Could you check a few things on this model? Use its own coordinates, in mm. A direction names the side the tool comes from. Give positions to 0.01 mm unless a question says otherwise; leave off trailing zeros. Write each loop counter-clockwise with the first axis right and the second up, starting at its lowest first coordinate (ties: lowest second). Pieces come first, ordered by that corner, then holes. Notation, with made-up numbers: (-22.75, 4.25) -> (22.25, 4.25) arc R22 ccw to (22.25, 36.25) -> close; hole circle Ø7 at (-32.75, 78.25). An arc over 180 degrees is marked (long way). One line per question, with ' | ' between items.
from build123d import *

# Parameters (mm, degrees)
SKETCH1_W           = 444.5
SKETCH1_H           = 285.75
BOSS_EXTRUDE1_DEPTH = 25.4
SKETCH2_R           = 6.7437
CUT_EXTRUDE1_DEPTH  = 530.035417056
SKETCH3_R           = 9.525
CUT_EXTRUDE2_DEPTH  = 7.62
SKETCH4_R           = 6.7437
CUT_EXTRUDE3_DEPTH  = 530.035417056


with BuildPart() as part:
    # Sketch1 → Boss-Extrude1 (new body)
    with BuildSketch(Plane.XY):
        with Locations((222.25, 142.875)):
            Rectangle(SKETCH1_W, SKETCH1_H)
    extrude(amount=BOSS_EXTRUDE1_DEPTH)

    # Sketch2 → Cut-Extrude1 (cut, through all)
    with BuildSketch(Plane.XY):
        with Locations((21.4376, 266.7)):
            Circle(SKETCH2_R)
        with Locations((423.0624, 266.7)):
            Circle(SKETCH2_R)
        with Locations((21.4376, 19.05)):
            Circle(SKETCH2_R)
        with Locations((423.0624, 19.05)):
            Circle(SKETCH2_R)
    extrude(amount=CUT_EXTRUDE1_DEPTH, mode=Mode.SUBTRACT)

    # Sketch3 → Cut-Extrude2 (cut)
    with BuildSketch(Plane.XY):
        with Locations(Location((21.4376, 266.7, 0), (0, 0, 180))):
            Circle(SKETCH3_R)
        with Locations(Location((423.0624, 266.7, 0), (0, 0, 180))):
            Circle(SKETCH3_R)
        with Locations(Location((21.4376, 19.05, 0), (0, 0, 180))):
            Circle(SKETCH3_R)
        with Locations(Location((423.0624, 19.05, 0), (0, 0, 180))):
            Circle(SKETCH3_R)
    extrude(amount=CUT_EXTRUDE2_DEPTH, mode=Mode.SUBTRACT)

    # Sketch4 → Cut-Extrude3 (cut, through all)
    with BuildSketch(Plane.XY):
        with Locations((193.675, 114.3)):
            Circle(SKETCH4_R)
        with Locations((371.475, 114.3)):
            Circle(SKETCH4_R)
        with Locations((193.675, 266.7)):
            Circle(SKETCH4_R)
        with Locations((371.475, 266.7)):
            Circle(SKETCH4_R)
    extrude(amount=CUT_EXTRUDE3_DEPTH, mode=Mode.SUBTRACT)


solid = part.part
Q1. Imagine slicing it at A-A on y = 114.3. Please give me the cut outline in (x, z), and give its area (3 significant figures).
Answer below:
outline: (0, 0) -> (186.93, 0) -> (186.93, 25.4) -> (0, 25.4) -> close; (200.42, 0) -> (364.73, 0) -> (364.73, 25.4) -> (200.42, 25.4) -> close; (378.22, 0) -> (444.5, 0) -> (444.5, 25.4) -> (378.22, 25.4) -> close | area: 10,600 mm^2
Q2. If we mould it in two halves opening along Y, with no side actions, what happens to faces 1 (the flat face through (430, 21, 7.62)), 2 (the flat face through (219, 0, 13)), 3 (the flat face through (219, 285.75, 13)), 4 (the cylindrical face through (22.678, 9.606, 3.757))? For each: +Y half, -Y half, draft (parallel to the pull), parting line (faces both ways), or undercut.
Answer below:
face 1: undercut | face 2: -Y half | face 3: +Y half | face 4: undercut
Q3. Imagine slicing it at C-C on y = 19.05. Please give me the cut outline in (x, z), and give its area (3 significant figures).
Answer below:
outline: (0, 0) -> (11.91, 0) -> (11.91, 7.62) -> (14.69, 7.62) -> (14.69, 25.4) -> (0, 25.4) -> close; (28.18, 7.62) -> (30.96, 7.62) -> (30.96, 0) -> (413.54, 0) -> (413.54, 7.62) -> (416.32, 7.62) -> (416.32, 25.4) -> (28.18, 25.4) -> close; (429.81, 7.62) -> (432.59, 7.62) -> (432.59, 0) -> (444.5, 0) -> (444.5, 25.4) -> (429.81, 25.4) -> close | area: 10,500 mm^2
Q4. Will these pins go through, and if not, where does the flat tip stop? pin 1 (21 mm diameter, centred on x = 423.5, y = 269.5, fed in from -Z); pin 2 (15 mm diameter, centred on x = 21.44, y = 266.7, fed in from -Z).
Answer below:
pin 1: stops at z = 0 | pin 2: stops at z = 7.62
Q5. If I drill on line 1 along X through (y, z) = (114.3, 6); line 2 along X through (y, z) = (266.7, 10); line 3 along X through (y, z) = (19.05, 19.5), over which ranges is the centre line in solid material (lowest first)?
Answer below:
line 1: x = 0 to 186.93, 200.42 to 364.73, 378.22 to 444.5 | line 2: x = 0 to 14.69, 28.18 to 186.93, 200.42 to 364.73, 378.22 to 416.32, 429.81 to 444.5 | line 3: x = 0 to 14.69, 28.18 to 416.32, 429.81 to 444.5
Q6. On a 3-axis mill with a long thin cutter (end or side, diameter ignored), from which of +Z, -Z, +X, -X, +Y, -Y can I reach the whole of each face in a straight line? I mean faces 5 (the cylindrical face through (16.086, 14.947, 16.386)), 6 (the flat face through (430, 269, 7.62)). Say none if no direction works.
Answer below:
face 5: +Z, -Z | face 6: -Z
Q7. Imagine slicing it at B-B on y = 266.7. Please give me the cut outline in (x, z), and give its area (3 significant figures).
Answer below:
outline: (0, 0) -> (11.91, 0) -> (11.91, 7.62) -> (14.69, 7.62) -> (14.69, 25.4) -> (0, 25.4) -> close; (28.18, 7.62) -> (30.96, 7.62) -> (30.96, 0) -> (186.93, 0) -> (186.93, 25.4) -> (28.18, 25.4) -> close; (200.42, 0) -> (364.73, 0) -> (364.73, 25.4) -> (200.42, 25.4) -> close; (378.22, 0) -> (413.54, 0) -> (413.54, 7.62) -> (416.32, 7.62) -> (416.32, 25.4) -> (378.22, 25.4) -> close; (429.81, 7.62) -> (432.59, 7.62) -> (432.59, 0) -> (444.5, 0) -> (444.5, 25.4) -> (429.81, 25.4) -> close | area: 9,840 mm^2
